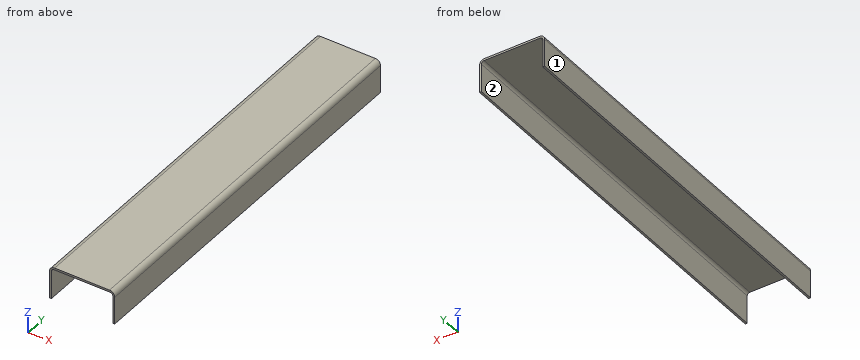
Autodesk Inventor part; units mm, degrees
ref_plane "YZ Plane" through (0, 0, 0) normal (1, 0, 0) x (0, 1, 0)
ref_plane "XZ Plane" through (0, 0, 0) normal (0, 1, 0) x (-1, 0, 0)
ref_plane "XY Plane" through (0, 0, 0) normal (0, 0, 1) x (1, 0, 0)
sketch "Sketch1" plane through (0, 0, 0) normal (0, 0, 1) x (1, 0, 0)
  line L0 (0, 53.34) -> (0, -53.34)
  line L1 (-8.89, 0) -> (8.89, 0)
  line L2 (-6.35, 38.1) -> (6.35, 38.1)
  line L3 (6.35, 38.1) -> (6.35, -38.1)
  line L4 (6.35, -38.1) -> (-6.35, -38.1)
  line L5 (-6.35, -38.1) -> (-6.35, 38.1)
  dimension "d0" = 12.7
  dimension "d1" = 76.2
extrude "Extrusion1" add sketch "Sketch1" along normal blind 6.35
shell "Shell1" thickness 0.381 removed faces 3 at (2.1167, -38.1, 2.1167) at (2.1167, -12.7, 0) at (-2.1167, 38.1, 2.1167)
fillet "Fillet1" radius 0.508 2 edges at (-5.969, 0, 5.969) (5.969, 0, 5.969)
fillet "Fillet1" radius 1.016 2 edges at (-6.35, 0, 6.35) (6.35, 0, 6.35)
properties part number "Staples" material "Steel, Mild"
Verification items for the finished model (mm, model axes). Face numbers are marked on the shaded views. A direction names the side the tool comes from. Coordinates: 2 decimals unless noted, no trailing zeros. Order: outer loops, then holes, each group sorted by start corner. A loop starts at its lowest first (then second) coordinate and runs counter-clockwise, first axis right, second up.
1. Go/stop test with flat-tipped pins: pin 1 Ø1 at (x, y) = (5, -11.5) entering from -Z; pin 2 Ø5 at (x, y) = (3.5, -11.5) entering from -Z. Record where each tip stops, or that it passes through.
Results found:
pin 1: stops at z = 5.97
pin 2: stops at z = 0
2. Scan lines: line 1 (X direction, y = -7, z = 2.75); line 2 (Z direction, x = -4.25, y = 30.5); line 3 (Z direction, x = 5.5, y = 15.5). Record each from-to range of solid material in increasing order.
Results found:
line 1: x = -6.35 to -5.97, 5.97 to 6.35
line 2: z = 5.97 to 6.35
line 3: z = 5.97 to 6.34
3. Set-up check for the marked faces 1 and 2: record each of +Z, -Z, +X, -X, +Y, -Y from which the full face is reachable in a straight line by a thin tool's end or side.
Results found:
face 1: +Z, -Z, -X, +Y, -Y
face 2: -Z, +Y, -Y
4. Sectioned sample at A-A, the plane z = 3.75. Record the cut outline in (x, y).
Results found:
outline: (-6.35, -38.1) - (-5.97, -38.1) - (-5.97, 38.1) - (-6.35, 38.1) - close; (5.97, -38.1) - (6.35, -38.1) - (6.35, 38.1) - (5.97, 38.1) - close
5. Sectioned sample at B-B, the plane y = -28.5. Record the cut outline in (x, z), and give its area (3 significant figures).
Results found:
outline: (-6.35, 0) - (-5.97, 0) - (-5.97, 5.46) arc R0.51 cw to (-5.46, 5.97) - (5.46, 5.97) arc R0.51 cw to (5.97, 5.46) - (5.97, 0) - (6.35, 0) - (6.35, 5.33) arc R1.02 ccw to (5.33, 6.35) - (-5.33, 6.35) arc R1.02 ccw to (-6.35, 5.33) - close
area: 9.05 mm2
6. Sectioned sample at C-C, the plane x = -3.75. Record the cut outline in (y, z).
Results found:
outline: (-38.1, 5.97) - (38.1, 5.97) - (38.1, 6.35) - (-38.1, 6.35) - close
